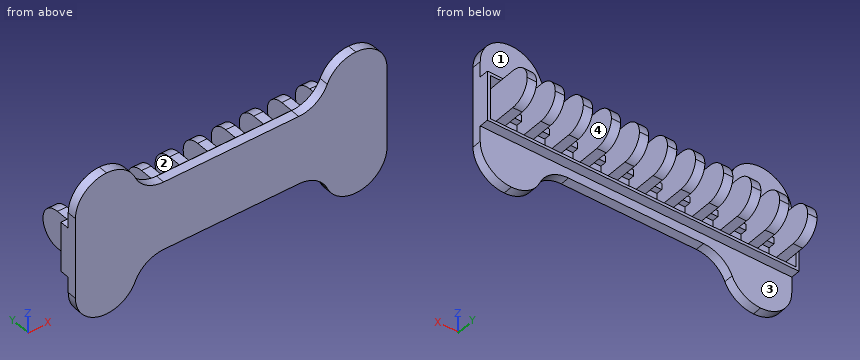
```python
from build123d import *

# Parameters (mm, degrees)
SKETCH1_W            = 100
SKETCH1_H            = 16
BOSS_EXTRUDE1_DEPTH  = 3
SKETCH2_W            = 98
SKETCH2_H            = 14
CUT_EXTRUDE1_DEPTH   = 1
SKETCH5_W            = 20
SKETCH5_H            = 3
BOSS_EXTRUDE4_DEPTH  = 15
SKETCH6_W            = 20
SKETCH6_H            = 3
BOSS_EXTRUDE5_DEPTH  = 15
FILLET18_R           = 10
SKETCH7_W            = 3
SKETCH7_H            = 12
BOSS_EXTRUDE6_DEPTH  = 16
SKETCH8_W            = 6
SKETCH8_H            = 2
BOSS_EXTRUDE7_DEPTH  = 2
FILLET19_R           = 6
SKETCH10_W           = 60
SKETCH10_H           = 3
BOSS_EXTRUDE8_DEPTH  = 3
SKETCH11_W           = 60
SKETCH11_H           = 3
BOSS_EXTRUDE9_DEPTH  = 3
SKETCH12_W           = 0.95
SKETCH12_H           = 14
BOSS_EXTRUDE10_DEPTH = 3
SKETCH13_W           = 100
SKETCH13_H           = 0.95
BOSS_EXTRUDE11_DEPTH = 3
SKETCH14_W           = 0.95
SKETCH14_H           = 0.052088128
BOSS_EXTRUDE12_DEPTH = 3
SKETCH15_W           = 0.95
SKETCH15_H           = 0.047911872
SKETCH15_W_2         = 0.949734752
SKETCH15_H_2         = 0.052088128
BOSS_EXTRUDE13_DEPTH = 3
FILLET20_R           = 10
SKETCH17_W           = 98.1
SKETCH17_H           = 14.1
SKETCH17_W_2         = 97.1
SKETCH17_H_2         = 13.1
CUT_EXTRUDE2_DEPTH   = 4


with BuildPart() as part:
    # Sketch1 → Boss-Extrude1 (new body)
    with BuildSketch(Plane(origin=(0, 0, 0), x_dir=(1, 0, 0), z_dir=(0, 1, 0))):
        with Locations((50, 8)):
            Rectangle(SKETCH1_W, SKETCH1_H)
    extrude(amount=BOSS_EXTRUDE1_DEPTH)

    # Sketch2 → Cut-Extrude1 (cut)
    with BuildSketch(Plane(origin=(0, 3, 0), x_dir=(1, 0, 0), z_dir=(0, 1, 0))):
        with Locations((50, 8)):
            Rectangle(SKETCH2_W, SKETCH2_H)
    extrude(amount=-CUT_EXTRUDE1_DEPTH, mode=Mode.SUBTRACT)

    # Sketch5 → Boss-Extrude4 (add)
    with BuildSketch(Plane.XY):
        with Locations((10, 1.5)):
            Rectangle(SKETCH5_W, SKETCH5_H)
        with Locations((90, 1.5)):
            Rectangle(SKETCH5_W, SKETCH5_H)
    extrude(amount=BOSS_EXTRUDE4_DEPTH)

    # Sketch6 → Boss-Extrude5 (add)
    with BuildSketch(Plane(origin=(0, 0, -16), x_dir=(-1, 0, 0), z_dir=(0, 0, -1))):
        with Locations((-90, 1.5)):
            Rectangle(SKETCH6_W, SKETCH6_H)
        with Locations((-10, 1.5)):
            Rectangle(SKETCH6_W, SKETCH6_H)
    extrude(amount=BOSS_EXTRUDE5_DEPTH)

    # Fillet18
    fillet18_edges = [part.edges().sort_by_distance(p)[0] for p in [
        (20, 1.5, 15),
        (0, 1.5, 15),
        (80, 1.5, 15),
        (100, 1.5, 15),
        (0, 1.5, -31),
        (20, 1.5, -31),
        (80, 1.5, -31),
        (100, 1.5, -31),
    ]]
    fillet(fillet18_edges, radius=FILLET18_R - 0.0001)  # a hair under: the kernel refuses the full size

    # Sketch7 → Boss-Extrude6 (add)
    with BuildSketch(Plane(origin=(0, 2, 0), x_dir=(1, 0, 0), z_dir=(0, 1, 0))):
        with Locations((95, 8)):
            Rectangle(SKETCH7_W, SKETCH7_H)
        with Locations((86, 8)):
            Rectangle(SKETCH7_W, SKETCH7_H)
        with Locations((77, 8)):
            Rectangle(SKETCH7_W, SKETCH7_H)
        with Locations((68, 8)):
            Rectangle(SKETCH7_W, SKETCH7_H)
        with Locations((59, 8)):
            Rectangle(SKETCH7_W, SKETCH7_H)
        with Locations((50, 8)):
            Rectangle(SKETCH7_W, SKETCH7_H)
        with Locations((41, 8)):
            Rectangle(SKETCH7_W, SKETCH7_H)
        with Locations((32, 8)):
            Rectangle(SKETCH7_W, SKETCH7_H)
        with Locations((23, 8)):
            Rectangle(SKETCH7_W, SKETCH7_H)
        with Locations((14, 8)):
            Rectangle(SKETCH7_W, SKETCH7_H)
        with Locations((5, 8)):
            Rectangle(SKETCH7_W, SKETCH7_H)
    extrude(amount=BOSS_EXTRUDE6_DEPTH)

    # Sketch8 → Boss-Extrude7 (add)
    with BuildSketch(Plane(origin=(0, 2, 0), x_dir=(1, 0, 0), z_dir=(0, 1, 0))):
        with Locations((90.5, 8)):
            Rectangle(SKETCH8_W, SKETCH8_H)
        with Locations((81.5, 8)):
            Rectangle(SKETCH8_W, SKETCH8_H)
        with Locations((72.5, 8)):
            Rectangle(SKETCH8_W, SKETCH8_H)
        with Locations((63.5, 8)):
            Rectangle(SKETCH8_W, SKETCH8_H)
        with Locations((54.5, 8)):
            Rectangle(SKETCH8_W, SKETCH8_H)
        with Locations((45.5, 8)):
            Rectangle(SKETCH8_W, SKETCH8_H)
        with Locations((36.5, 8)):
            Rectangle(SKETCH8_W, SKETCH8_H)
        with Locations((27.5, 8)):
            Rectangle(SKETCH8_W, SKETCH8_H)
        with Locations((18.5, 8)):
            Rectangle(SKETCH8_W, SKETCH8_H)
        with Locations((9.5, 8)):
            Rectangle(SKETCH8_W, SKETCH8_H)
    extrude(amount=BOSS_EXTRUDE7_DEPTH)

    # Fillet19
    fillet19_edges = [part.edges().sort_by_distance(p)[0] for p in [
        (95, 18, -2),
        (95, 18, -14),
        (86, 18, -2),
        (86, 18, -14),
        (77, 18, -2),
        (77, 18, -14),
        (68, 18, -2),
        (68, 18, -14),
        (59, 18, -2),
        (59, 18, -14),
        (50, 18, -2),
        (50, 18, -14),
        (41, 18, -2),
        (41, 18, -14),
        (32, 18, -2),
        (32, 18, -14),
        (23, 18, -14),
        (23, 18, -2),
        (14, 18, -2),
        (14, 18, -14),
        (5, 18, -2),
        (5, 18, -14),
    ]]
    fillet(fillet19_edges, radius=FILLET19_R - 0.0001)  # a hair under: the kernel refuses the full size

    # Sketch10 → Boss-Extrude8 (add)
    with BuildSketch(Plane(origin=(0, 0, -16), x_dir=(-1, 0, 0), z_dir=(0, 0, -1))):
        with Locations((-50, 1.5)):
            Rectangle(SKETCH10_W, SKETCH10_H)
    extrude(amount=BOSS_EXTRUDE8_DEPTH)

    # Sketch11 → Boss-Extrude9 (add)
    with BuildSketch(Plane.XY):
        with Locations((50, 1.5)):
            Rectangle(SKETCH11_W, SKETCH11_H)
    extrude(amount=BOSS_EXTRUDE9_DEPTH)

    # Sketch12 → Boss-Extrude10 (add)
    with BuildSketch(Plane(origin=(0, 3, 0), x_dir=(1, 0, 0), z_dir=(0, 1, 0))):
        with Locations((99.525, 7.997911872)):
            Rectangle(SKETCH12_W, SKETCH12_H)
        with Locations((0.475, 7.997911872)):
            Rectangle(SKETCH12_W, SKETCH12_H)
    extrude(amount=BOSS_EXTRUDE10_DEPTH)

    # Sketch13 → Boss-Extrude11 (add)
    with BuildSketch(Plane(origin=(0, 3, 0), x_dir=(1, 0, 0), z_dir=(0, 1, 0))):
        with Locations((50, 15.525)):
            Rectangle(SKETCH13_W, SKETCH13_H)
        with Locations((50, 0.475)):
            Rectangle(SKETCH13_W, SKETCH13_H)
    extrude(amount=BOSS_EXTRUDE11_DEPTH)

    # Sketch14 → Boss-Extrude12 (add)
    with BuildSketch(Plane(origin=(0, 3, 0), x_dir=(1, 0, 0), z_dir=(0, 1, 0))):
        with Locations((0.475, 15.023955936)):
            Rectangle(SKETCH14_W, SKETCH14_H)
    extrude(amount=BOSS_EXTRUDE12_DEPTH)

    # Sketch15 → Boss-Extrude13 (add)
    with BuildSketch(Plane(origin=(0, 3, 0), x_dir=(1, 0, 0), z_dir=(0, 1, 0))):
        with Locations((0.475, 0.973955936)):
            Rectangle(SKETCH15_W, SKETCH15_H)
        with Locations((99.525132624, 0.973955936)):
            Rectangle(SKETCH15_W_2, SKETCH15_H)
        with Locations((99.525, 15.023955936)):
            Rectangle(SKETCH15_W, SKETCH15_H_2)
    extrude(amount=BOSS_EXTRUDE13_DEPTH)

    # Fillet20
    fillet20_edges = [part.edges().sort_by_distance(p)[0] for p in [
        (20, 1.5, -19),
        (80, 1.5, -19),
        (80, 1.5, 3),
        (20, 1.5, 3),
    ]]
    fillet(fillet20_edges, radius=FILLET20_R)

    # Sketch17 → Cut-Extrude2 (cut)
    with BuildSketch(Plane(origin=(0, 6, 0), x_dir=(1, 0, 0), z_dir=(0, 1, 0))):
        with Locations((50, 8)):
            Rectangle(SKETCH17_W, SKETCH17_H)
        with Locations((50, 8)):
            Rectangle(SKETCH17_W_2, SKETCH17_H_2, mode=Mode.SUBTRACT)
    extrude(amount=-CUT_EXTRUDE2_DEPTH, mode=Mode.SUBTRACT)


solid = part.part
```
The listing builds one solid part. Answer for the finished solid, in the listing's coordinates (mm). Face numbers are marked on the shaded views. A direction names the side the tool comes from. Coordinates: 2 decimals unless noted, no trailing zeros. Write each loop counter-clockwise with the first axis right and the second up, starting at its lowest first coordinate (ties: lowest second). Pieces come first, ordered by that corner, then holes. Notation, with made-up numbers: (46.5, 40.5) - (58.5, 40.5) arc R23 ccw to (58.5, 54.5) - close; hole circle Ø6 at (82, 36). An arc over 180 degrees is marked (long way). Return JSON: item names as keys, results as strings. Group by question number.
1. A cutting plane is placed at A-A, the plane x = 37. Determine the outline of the cut face in (y, z).
2. A cutting plane is placed at B-B, the plane y = 10.5. Give the number of separate pieces and of enclosed holes in the cut face, plus the area to 3 significant figures.
3. Determine the mould class of the marked faces 3 and 4 for opening direction Z: released by +Z, released by -Z, zero draft, split by the parting line, or undercut.
4. A cutting plane is placed at C-C, the plane x = 9. Determine the outline of the cut face in (y, z), plus the area to 3 significant figures.
5. Which of the six approach directions +Z, -Z, +X, -X, +Y, -Y give full straight-line access (tool end or side, diameter ignored) to the marked faces 1 and 2?
6. Given pin 1 (4 mm diameter, centred on x = 11, z = -10.5, fed in from +Y); pin 2 (3.5 mm diameter, centred on x = 13.5, y = 8.5, fed in from -Z); pin 3 (4.5 mm diameter, centred on x = 54, y = 3, fed in from +Z), each flat-ended and moving along its own axis, determine where each tip first touches the part or whether it passes through.
7. Straight lines are drawn through the part: L1, parallel to Z at x = 72, y = 2.75; L2, parallel to Z at x = 29, y = 3.5; L3, parallel to Y at x = 71.5, z = -14. For each, find the intervals that lie inside material, in ascending order.
Ans:
{
 "1": {"outline": "(0, -19) - (3, -19) - (3, -16) - (6, -16) - (6, -15.05) - (2, -15.05) - (2, -9) - (4, -9) - (4, -7) - (2, -7) - (2, -0.95) - (6, -0.95) - (6, 0) - (3, 0) - (3, 3) - (0, 3) - close"},
 "2": {"separate pieces": "11", "enclosed holes": "0", "area": "396 mm²"},
 "3": {"face 3": "zero draft", "face 4": "undercut"},
 "4": {"outline": "(0, -30.95) - (3, -30.95) - (3, -16) - (6, -16) - (6, -15.05) - (2, -15.05) - (2, -9) - (4, -9) - (4, -7) - (2, -7) - (2, -0.95) - (6, -0.95) - (6, 0) - (3, 0) - (3, 14.95) - (0, 14.95) - close", "area": "133 mm²"},
 "5": {"face 1": "+Z, +X, -X, +Y", "face 2": "+Y"},
 "6": {"pin 1": "y = 17.88", "pin 2": "z = -14", "pin 3": "z = 3"},
 "7": {"L1": "-19.01 to -15.05, -9 to -7, -0.95 to 3.01", "L2": "-16 to -15.05, -9 to -7, -0.95 to 0", "L3": "0 to 2"}
}
